Print and shaded views of the part. All mm, measured from the part's lowest x, y and z. A direction names the side the tool comes from. Give positions to 0.01 mm unless a question says otherwise; leave off trailing zeros. Order: outer loops, then holes, each group sorted by start corner. A loop starts at its lowest first (then second) coordinate and runs counter-clockwise, first axis right, second up. Notation, with made-up numbers: (63.25, -16.5) -> (102.25, -16.5) arc R29 ccw to (102.25, 17.5) -> close; hole circle Ø3 at (58.25, -33.5). An arc over 180 degrees is marked (long way). One line per question, with ' | ' between items. Start each with the question number.
(1) Cut at C-C (x = 8.5). Give the number of separate pieces and of enclosed holes in the cut face, then the cut area to 3 significant figures.
(2) Drill centre lines: L1, parallel to Z at x = 3.5, y = 12; L2, parallel to Z at x = 9, y = 3.5 (1 decimal); L3, parallel to Z at x = 6.9, y = 27.1 (1 decimal). Where is each one in solid material? Low to high. Write a range as from..to.
(3) Pull direction Z, two halves, no side cores. Call the marked faces 5, 6, 7 and 8: +Z half, -Z half, draft (parallel to the pull), parting line (faces both ways), or undercut.
(4) Cut at B-B (y = 26.5). Give the cut face in (x, z).
(5) Which spindle directions (+Z, -Z, +X, -X, +Y, -Y) get a long thin tool onto all of the face, cutting with end or side? Do the marked faces 1, 2, 3 and 4. Say none if no direction does.
(6) Pin check, flat tips, straight feed: pin 1 Ø5 at (x, z) = (6, 18) entering from +Y; pin 2 Ø3 at (y, z) = (4.1, 27.1) entering from -X; pin 3 Ø5.5 at (x, y) = (1.5, 16.5) entering from -Z; pin 4 Ø5 at (x, y) = (6, 7) entering from +Z. Stop position of each tip, or through.
(7) Cut at D-D (y = 18). Give the cut face in (x, z).
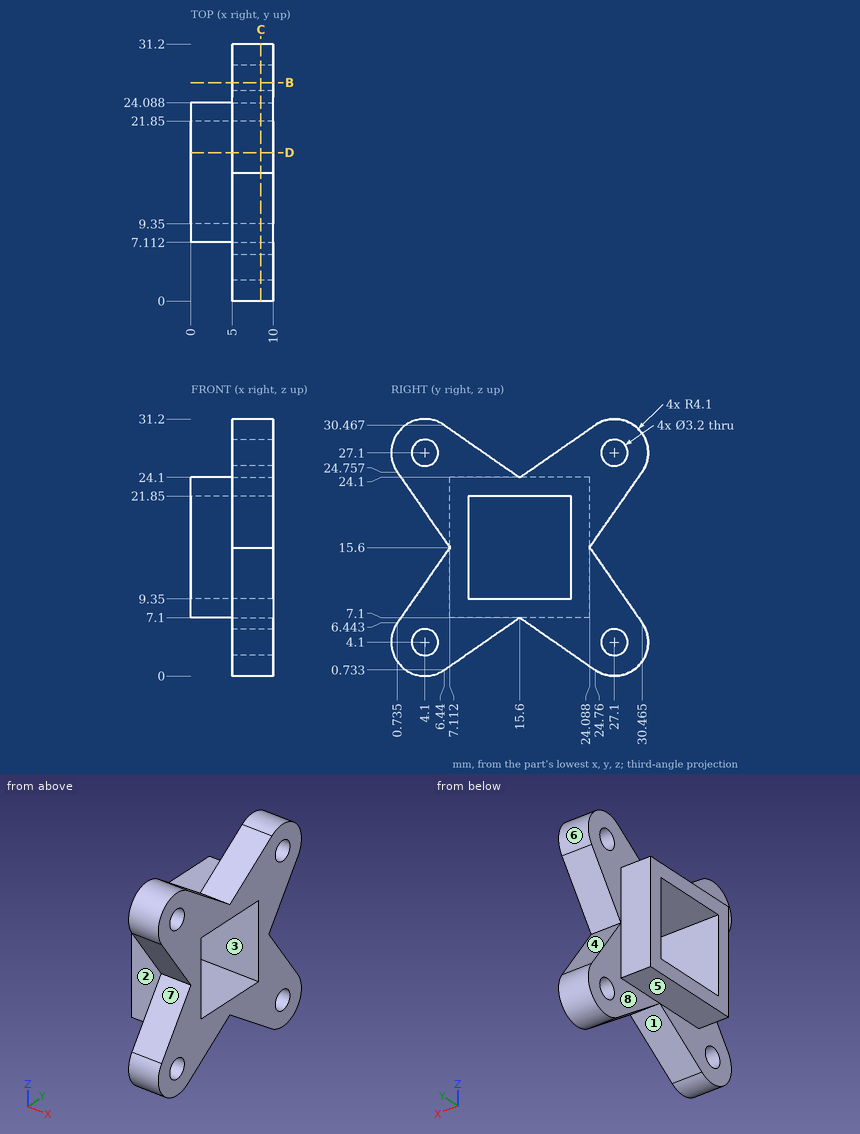
Result set:
1) separate pieces: 1 | enclosed holes: 5 | area: 479 mm2
2) L1: z = 7.1..9.35, 21.85..24.1 | L2: z = 0..2.6, 5.6..10.4, 20.8..25.6, 28.6..31.2 | L3: z = 0..2.5, 5.7..11.3, 19.9..25.5, 28.7..31.2
3) face 5: -Z half | face 6: undercut | face 7: undercut | face 8: draft
4) outline: (5, 0.04) -> (10, 0.04) -> (10, 2.62) -> (5, 2.62) -> close; (5, 5.58) -> (10, 5.58) -> (10, 12.14) -> (5, 12.14) -> close; (5, 19.06) -> (10, 19.06) -> (10, 25.62) -> (5, 25.62) -> close; (5, 28.58) -> (10, 28.58) -> (10, 31.16) -> (5, 31.16) -> close
5) face 1: -Z, +X, -X | face 2: +Z, -Z, -X, -Y | face 3: +X, -X | face 4: +X, -X, +Y
6) pin 1: stops at y = 27.5 | pin 2: passes through | pin 3: stops at z = 7.1 | pin 4: stops at z = 31.18
7) outline: (0, 7.1) -> (5, 7.1) -> (5, 5.43) -> (10, 5.43) -> (10, 9.35) -> (0, 9.35) -> close; (0, 21.85) -> (10, 21.85) -> (10, 25.77) -> (5, 25.77) -> (5, 24.1) -> (0, 24.1) -> close
